Can you work these out from the model? Positions are in its coordinate system, mm. Round coordinates to 2 decimals unless told otherwise and drop trailing zeros. Loops run counter-clockwise (first coordinate to the right, second up) from the corner with the lowest first, then second, coordinate; pieces in that order, holes last.
(1) Will these pins go through, and if not, where does the flat tip stop? pin 1 Ø12.5 at (x, z) = (-175.78, -90.12) entering from +Y; pin 2 Ø8.5 at (x, z) = (90.92, -13.92) entering from -Y; pin 3 Ø4 at (x, y) = (-20.5, -4) entering from -Z.
(2) I want a section at A-A on x = 19. Write out the boundary of the cut face in (y, z).
(3) If I drill on line 1 along X through (y, z) = (-4.25, -15); line 2 along Z through (x, y) = (89.5, -14.5); line 3 along X through (y, z) = (-1, -83), over which ranges is the centre line in solid material (lowest first)?
(4) I want a section at C-C on z = 54. Write out the boundary of the cut face in (x, y), plus the area to 3 significant figures.
(5) I want a section at B-B on y = -4. Give the number of separate pieces and of enclosed holes in the cut face, plus the area to 3 significant figures.
from build123d import *

# Parameters (mm, degrees)
F0_W           = 304.8
F0_H           = 203.2
F1_DEPTH       = 19.05
F2_W           = 228.6
F2_H           = 23.8541702911
F3_DEPTH       = 19.051
F4_R           = 6.35
F5_R           = 6.35
F6_DEPTH       = 12.7
F8_D           = 9.525
F8_CBORE_D     = 15.875
F8_CBORE_DEPTH = 12.7
F9_SIZE        = 50.8


with BuildPart() as f1:
    # F0 (on Front) → F1 (new body)
    with BuildSketch(Plane.XZ):
        with Locations((-42.4302353088, -7.5749112293)):
            Rectangle(F0_W, F0_H)
    extrude(amount=F1_DEPTH)

    # F2 (on face) → F3 (cut, through all)
    with BuildSketch(Plane.XZ.offset(19.05)):
        with Locations((-42.4302353088, -97.2478260837)):
            Rectangle(F2_W, F2_H)
    extrude(amount=-F3_DEPTH, mode=Mode.SUBTRACT)

    # F4
    f4_edges = [f1.edges().sort_by_distance(p)[0] for p in [
        (-156.730235, -9.525, -85.320741),
        (-156.730235, -9.525, -109.174911),
        (-194.830235, -9.525, -109.174911),
        (71.869765, -9.525, -85.320741),
        (71.869765, -9.525, -109.174911),
        (109.969765, -9.525, -109.174911),
    ]]
    fillet(f4_edges, radius=F4_R)

    # F5 (on face) → F6 (cut)
    with BuildSketch(Plane(origin=(0, 0, 0), x_dir=(-1, 0, 0), z_dir=(0, 1, 0))):
        with Locations((-84.5697646912, 23.4674590618)):
            Circle(F5_R)
        with BuildLine():
            ThreePointArc((175.7802353088, 23.4674590618), (169.4302353088, 29.8174590618), (163.0802353088, 23.4674590618))
            ThreePointArc((163.0802353088, 23.4674590618), (169.4302353088, 17.1174590618), (175.7802353088, 23.4674590618))
        make_face()
    extrude(amount=-F6_DEPTH, mode=Mode.SUBTRACT)

    # F8 (through all)
    with Locations(Plane(origin=(0, 0, 0), x_dir=(-1, 0, 0), z_dir=(0, 1, 0))):
        with Locations((-90.9197646912, -13.9249112293), (-90.9197646912, -90.1249112293), (175.7802353088, -90.1249112293), (175.7802353088, -13.9249112293)):
            CounterBoreHole(F8_D / 2, F8_CBORE_D / 2, F8_CBORE_DEPTH)

    # F9
    f9_edges = [f1.edges().sort_by_distance(p)[0] for p in [
        (109.969765, -9.525, 94.025089),
        (-194.830235, -9.525, 94.025089),
    ]]
    chamfer(f9_edges, length=F9_SIZE)


solid = f1.part
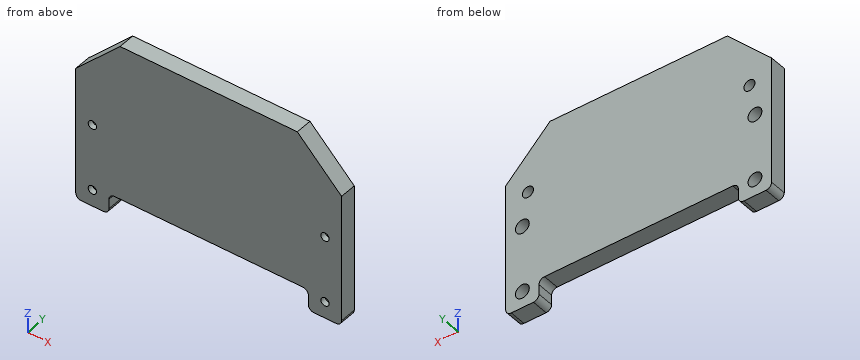
Filled sheet:
1. pin 1: stops at y = -12.7
1. pin 2: passes through
1. pin 3: stops at z = -85.32
2. outline: (-19.05, -85.32) - (0, -85.32) - (0, 94.03) - (-19.05, 94.03) - close
3. line 1: x = -194.83 to -183.64, -167.92 to 83.06, 98.78 to 109.97
3. line 2: z = -109.17 to -94.67, -85.58 to -18.47, -9.38 to 63.69
3. line 3: x = -194.83 to -179.28, -172.28 to 87.42, 94.42 to 109.97
4. outline: (-184.06, -19.05) - (99.19, -19.05) - (99.19, 0) - (-184.06, 0) - close
4. area: 5,400 mm2
5. separate pieces: 1
5. enclosed holes: 6
5. area: 52,800 mm2
